from build123d import *

# Parameters (mm, degrees)
ESQUISSE1_W        = 230
ESQUISSE1_H        = 58
ESQUISSE1_R        = 1.75
BOSS_EXTRU_1_DEPTH = 10


with BuildPart() as part:
    # Esquisse1 → Boss.-Extru.1 (new body)
    with BuildSketch(Plane.XY):
        with Locations((-19.287380446, 0.978440775)):
            Rectangle(ESQUISSE1_W, ESQUISSE1_H)
        with Locations((83.712619554, 19.978440775)):
            Circle(ESQUISSE1_R, mode=Mode.SUBTRACT)
        with Locations((66.712619554, -23.021559225)):
            Circle(ESQUISSE1_R, mode=Mode.SUBTRACT)
        with BuildLine():
            Line((-114.287380446, 9.978440775), (45.712619554, 9.978440775))
            ThreePointArc((45.712619554, 9.978440775), (54.712619554, 0.978440775), (45.712619554, -8.021559225))
            Line((45.712619554, -8.021559225), (-114.287380446, -8.021559225))
            ThreePointArc((-114.287380446, -8.021559225), (-123.287380446, 0.978440775), (-114.287380446, 9.978440775))
        make_face(mode=Mode.SUBTRACT)
    extrude(amount=BOSS_EXTRU_1_DEPTH)


solid = part.part
Geometry: final body of the model. Coordinates: model frame, mm. A direction names the side the tool comes from. Give positions to 0.01 mm unless a question says otherwise; leave off trailing zeros. Loops run counter-clockwise (first coordinate to the right, second up) from the corner with the lowest first, then second, coordinate; pieces in that order, holes last. Notation, with made-up numbers: (53.25, -13.5) - (92.25, -13.5) arc R18 cw to (92.25, 12.5) - close; hole circle Ø11 at (36.5, 86.25). An arc over 180 degrees is marked (long way). One line per question, with ' | ' between items. Start each with the question number.
(1) Section query A-A on x = -63. Return loops of the section in (y, z), then the cut area to 3 significant figures.
(2) Pull-direction query (Y, two-part tool) for faces 3 (the flat face through (-35, 9.978, 5)), 4 (the flat face through (-21, -28.022, 5)), 5 (the flat face through (-21, 14, 0)); classes: released by +Y, released by -Y, zero draft, split by the parting line, or undercut.
(3) Ray query, line 1 (Y direction, x = -113, z = 3); line 2 (X direction, y = 1.5, z = 3.5); line 3 (X direction, y = 18.5, z = 2.25). Return the intervals inside material, ascending. Write a range as from..to.
(4) Reachability of faces 1 (the flat face through (-134.287, 1, 5)), 2 (the cylindrical face through (-123.285, 0.781, 4.93)) from +Z, -Z, +X, -X, +Y, -Y: full face, straight path, thin tool, end or side. Return the list, or none.
(5) Section query B-B on y = -4.5. Return loops of the section in (x, z).
(6) Section query C-C on z = 7.25. Return loops of the section in (x, y), then the cut area to 3 significant figures.
The answers:
1) outline: (-28.02, 0) - (-8.02, 0) - (-8.02, 10) - (-28.02, 10) - close; (9.98, 0) - (29.98, 0) - (29.98, 10) - (9.98, 10) - close | area: 400 mm2
2) face 3: undercut | face 4: released by -Y | face 5: zero draft
3) line 1: -28.02..-8.02, 9.98..29.98 | line 2: -134.29..-123.27, 54.7..95.71 | line 3: -134.29..82.78, 84.65..95.71
4) face 1: +Z, -Z, -X, +Y, -Y | face 2: +Z, -Z
5) outline: (-134.29, 0) - (-121.43, 0) - (-121.43, 10) - (-134.29, 10) - close; (52.85, 0) - (95.71, 0) - (95.71, 10) - (52.85, 10) - close
6) outline: (-134.29, -28.02) - (95.71, -28.02) - (95.71, 29.98) - (-134.29, 29.98) - close; hole (-114.29, -8.02) - (45.71, -8.02) arc R9 ccw to (45.71, 9.98) - (-114.29, 9.98) arc R9 ccw to start; hole circle Ø3.5 at (66.71, -23.02); hole circle Ø3.5 at (83.71, 19.98) | area: 10,200 mm2
